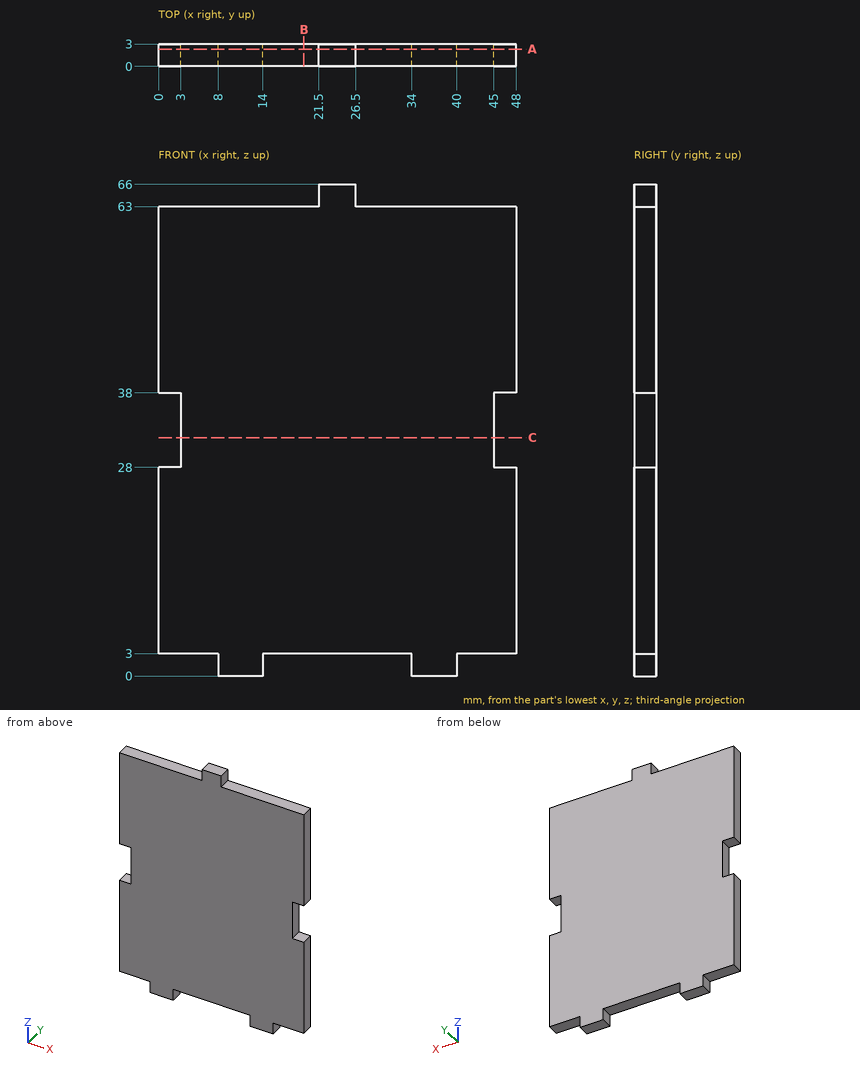
Can you work these out from the drawing? Everything is in mm from the part's minimum corner. Give positions to 0.01 mm unless a question says otherwise; leave off trailing zeros. Order: outer loops, then holes, each group sorted by start corner. A loop starts at its lowest first (then second) coordinate and runs counter-clockwise, first axis right, second up. Notation, with made-up numbers: (74, -7) -> (122, -7) arc R19 ccw to (122, 17) -> close; hole circle Ø10 at (-20, -15.5). An arc over 180 degrees is marked (long way). Return JSON: item names as keys, results as strings.
1. Imagine slicing it at B-B on x = 19.5. List the corners of the cut face in (y, z) for me, then the cut area to 3 significant figures.
Answer list:
{"outline": "(0, 3) -> (3, 3) -> (3, 63) -> (0, 63) -> close", "area": "180 mm2"}
2. Imagine slicing it at C-C on z = 32. List the corners of the cut face in (x, y) for me, then the cut area to 3 significant figures.
Answer list:
{"outline": "(3, 0) -> (45, 0) -> (45, 3) -> (3, 3) -> close", "area": "126 mm2"}
3. I need wall thicknesses on line 1 (Z direction, x = 15.5, y = 1.1); line 2 (X direction, y = 2.45, z = 33); line 3 (Z direction, x = 39, y = 1). Which ranges of each line are inside material? Lowest first, please. Write a range as from..to.
Answer list:
{"line 1": "z = 3..63", "line 2": "x = 3..45", "line 3": "z = 0..63"}
4. For pin 1 Ø0.9 at (y, z) = (1.5, 1.5) entering from -X; pin 2 Ø0.9 at (x, y) = (29, 1.5) entering from -Z; pin 3 Ø0.9 at (y, z) = (1.5, 1.5) entering from +X, each with a flat end and sliding along its axis, tell me the tip position at first contact or that it passes through.
Answer list:
{"pin 1": "stops at x = 8", "pin 2": "stops at z = 3", "pin 3": "stops at x = 40"}
5. Imagine slicing it at A-A on y = 2.3. List the corners of the cut face in (x, z) for me.
Answer list:
{"outline": "(0, 3) -> (8, 3) -> (8, 0) -> (14, 0) -> (14, 3) -> (34, 3) -> (34, 0) -> (40, 0) -> (40, 3) -> (48, 3) -> (48, 28) -> (45, 28) -> (45, 38) -> (48, 38) -> (48, 63) -> (26.5, 63) -> (26.5, 66) -> (21.5, 66) -> (21.5, 63) -> (0, 63) -> (0, 38) -> (3, 38) -> (3, 28) -> (0, 28) -> close"}
